Verification items for the finished model (mm, model axes). Give positions to 0.01 mm unless a question says otherwise; leave off trailing zeros. Write each loop counter-clockwise with the first axis right and the second up, starting at its lowest first coordinate (ties: lowest second). Pieces come first, ordered by that corner, then holes.
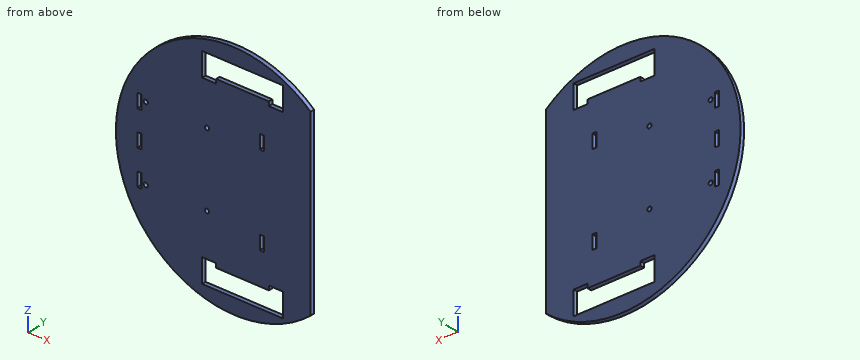
Autodesk Inventor part; units mm, degrees
ref_plane "YZ Plane" through (0, 0, 0) normal (1, 0, 0) x (0, 1, 0)
ref_plane "XZ Plane" through (0, 0, 0) normal (0, 1, 0) x (-1, 0, 0)
ref_plane "XY Plane" through (0, 0, 0) normal (0, 0, 1) x (1, 0, 0)
sketch "Sketch1" plane through (0, 0, 0) normal (0, 1, 0) x (-1, 0, 0)
  circle A0 centre (0, 0) radius 85 construction
  line L0 (-55, 64.8074) -> (-55, -64.8074) construction
  line L1 (-35, 74) -> (23, 74) construction
  line L2 (23, 74) -> (23, 60) construction
  line L3 (23, 60) -> (-35, 60) construction
  line L4 (-35, 60) -> (-35, 74) construction
  line L5 (-35, -60) -> (23, -60) construction
  line L6 (23, -60) -> (23, -74) construction
  line L7 (23, -74) -> (-35, -74) construction
  line L8 (-35, -74) -> (-35, -60) construction
  line L9 (-6, 60) -> (-6, -60)
  line L10 (6.5, 5) -> (-18.5, 5) construction
  line L11 (-18.5, 5) -> (-18.5, 57) construction
  line L12 (-18.5, 57) -> (6.5, 57) construction
  line L13 (6.5, 57) -> (6.5, 5) construction
  line L14 (6.5, 5) -> (-18.5, 57) construction
  line L15 (-18.5, 5) -> (6.5, 57) construction
  line L16 (6.5, -57) -> (-18.5, -57) construction
  line L17 (-18.5, -57) -> (-18.5, -5) construction
  line L18 (-18.5, -5) -> (6.5, -5) construction
  line L19 (6.5, -5) -> (6.5, -57) construction
  line L20 (6.5, -57) -> (-18.5, -5) construction
  line L21 (-18.5, -57) -> (6.5, -5) construction
  line L22 (66.5, -30) -> (16.5, -30) construction
  line L23 (16.5, -30) -> (16.5, 30) construction
  line L24 (16.5, 30) -> (66.5, 30) construction
  line L25 (66.5, 30) -> (66.5, -30) construction
  line L26 (66.5, -30) -> (16.5, 30) construction
  line L27 (16.5, -30) -> (66.5, 30) construction
  point P0 (-6, 31)
  point P1 (-6, -31)
  point P2 (41.5, 0)
  point P3 (-6, 0)
  point P4 (41.5, 0)
  dimension "d0" = 170
  dimension "d1" = 55
  dimension "d2" = 58
  dimension "d3" = 14
  dimension "d4" = 60
  dimension "d5" = 20
  dimension "d6" = 60
  dimension "d7" = 25
  dimension "d8" = 52
  dimension "d9" = 3
  dimension "d10" = 3
  dimension "d11" = 10
  dimension "d12" = 50
  dimension "d13" = 60
  dimension "d14" = 10
sketch "Sketch2" plane through (0, 0, 0) normal (0, 1, 0) x (-1, 0, 0)
  circle A0 centre (0, 0) radius 85 construction
  line L0 (-55, 64.8074) -> (-55, -64.8074) construction
  arc A1 (-55, -64.8074) -> (-55, 64.8074) centre (0, 0) ccw
  line L1 (-55, 64.8074) -> (-55, -64.8074)
extrude "Extrusion1" add sketch "Sketch2" along normal blind 3
sketch "Sketch3" plane through (0, 0, 0) normal (0, -1, 0) x (1, 0, 0)
  line L0 (-23, 74) -> (35, 74)
  line L1 (35, 74) -> (35, 60)
  line L2 (35, 60) -> (-23, 60)
  line L3 (-23, 60) -> (-23, 74)
  point P0 (0, 0)
extrude "Extrusion2" cut sketch "Sketch3" against normal blind 3
sketch "Sketch4" plane through (0, 0, 0) normal (0, -1, 0) x (1, 0, 0)
  line L0 (-23, 60) -> (-13, 60)
  line L1 (-13, 60) -> (-13, 57)
  line L2 (-13, 57) -> (-23, 57)
  line L3 (-23, 57) -> (-23, 60)
  line L4 (35, 60) -> (25, 60)
  line L5 (25, 60) -> (25, 57)
  line L6 (25, 57) -> (35, 57)
  line L7 (35, 57) -> (35, 60)
  point P0 (0, 0)
  dimension "d19" = 10
  dimension "d20" = 3
  dimension "d21" = 10
  dimension "d22" = 3
extrude "Extrusion3" cut sketch "Sketch4" against normal blind 3
sketch "Sketch5" plane through (0, 0, 0) normal (0, -1, 0) x (1, 0, 0)
  line L0 (18.5, 5) -> (18.5, 57) construction
  line L1 (18.5, 37) -> (21.5, 37)
  line L2 (21.5, 37) -> (21.5, 27)
  line L3 (21.5, 27) -> (18.5, 27)
  line L4 (18.5, 27) -> (18.5, 37)
  line L5 (35, 57) -> (25, 57)
  point P0 (0, 0)
  dimension "d25" = 3
  dimension "d26" = 10
  dimension "d27" = 20
extrude "Extrusion4" cut sketch "Sketch5" against normal blind 3
sketch "Sketch6" plane through (0, 0, 0) normal (0, -1, 0) x (1, 0, 0)
  line L0 (-66.5, 30) -> (-66.5, -30) construction
  line L1 (-66.5, 30) -> (-69.5, 30)
  line L2 (-69.5, 30) -> (-69.5, 20)
  line L3 (-69.5, 20) -> (-66.5, 20)
  line L4 (-66.5, 20) -> (-66.5, 30)
  line L5 (-66.5, 5) -> (-69.5, 5)
  line L6 (-69.5, 5) -> (-69.5, -5)
  line L7 (-69.5, -5) -> (-66.5, -5)
  line L8 (-66.5, -5) -> (-66.5, 5)
  line L9 (-66.5, -30) -> (-69.5, -30)
  line L10 (-69.5, -30) -> (-69.5, -20)
  line L11 (-69.5, -20) -> (-66.5, -20)
  line L12 (-66.5, -20) -> (-66.5, -30)
  point P0 (0, 0)
  point P1 (-69.5, 0)
  point P2 (-66.5, 0)
  dimension "d30" = 3
  dimension "d31" = 10
  dimension "d32" = 3
  dimension "d33" = 10
  dimension "d34" = 3
  dimension "d35" = 10
extrude "Extrusion5" cut sketch "Sketch6" against normal blind 3
sketch "Sketch7" plane through (0, 0, 0) normal (0, -1, 0) x (1, 0, 0)
  line L0 (-16.5, -30) -> (-66.5, 30) construction
  line L1 (-63.5, 26.4) -> (-19.5, 26.4)
  line L2 (-19.5, 26.4) -> (-19.5, -26.4)
  line L3 (-19.5, -26.4) -> (-63.5, -26.4)
  line L4 (-63.5, -26.4) -> (-63.5, 26.4)
  line L5 (-63.5, 26.4) -> (-19.5, -26.4) construction
  line L6 (-19.5, 26.4) -> (-63.5, -26.4) construction
  line L7 (-16.5, -30) -> (-16.5, 30) construction
  circle A0 centre (-19.5, 26.4) radius 1.5
  circle A1 centre (-19.5, -26.4) radius 1.5
  circle A2 centre (-63.5, 26.4) radius 1.5
  circle A3 centre (-63.5, -26.4) radius 1.5
  point P0 (0, 0)
  point P1 (-41.5, 0)
  dimension "d38" = 3
  dimension "d39" = 3
  dimension "d40" = 3
  dimension "d41" = 3
  dimension "d42" = 3
extrude "Extrusion6" cut sketch "Sketch7" against normal blind 3 contours L4 A2 L1 | L1 A2 L4 | A0 L2 L1 | L1 L2 A0
mirror "Mirror1" about plane through (0, 0, 0) normal (0, 0, 1) of "Extrusion2", "Extrusion3", "Extrusion4", "Extrusion6"
equation "\"d10\" = d9"
properties part number "Base Plate"
Item 1: Sectioned sample at B-B on y = 2.55. State how many separate pieces and enclosed holes the cut face has, then the cut area to 3 significant figures.
Answer key:
separate pieces: 1
enclosed holes: 11
area: 18,100 mm2
Item 2: Sectioned sample at C-C on x = 40. Record the cut outline in (y, z).
Answer key:
outline: (0, -75) - (3, -75) - (3, 75) - (0, 75) - close
Item 3: Depth check by flat-ended pin: pin 1 (1.5 mm diameter, centred on x = 32.5, y = 1, fed in from -Z); pin 2 (0.9 mm diameter, centred on x = 20.5, y = 1, fed in from +Z); pin 3 (5 mm diameter, centred on x = -8, z = 29, fed in from -Y); pin 4 (1.8 mm diameter, centred on x = -19.5, z = 26.4, fed in from -Y). Enter the tip coordinate at first touch or a pass-through.
Answer key:
pin 1: stops at z = -78.85
pin 2: stops at z = 82.6
pin 3: stops at y = 0
pin 4: passes through
Item 4: Scan lines: line 1 along Z through (x, y) = (0, 1.1); line 2 along X through (y, z) = (1.2, 26.4); line 3 along Z through (x, y) = (-19.5, 1). Record each from-to range of solid material in increasing order.
Answer key:
line 1: z = -85 to -74, -60 to 60, 74 to 85
line 2: x = -80.8 to -69.5, -66.5 to -65, -62 to -21, -18 to 55
line 3: z = -82.73 to -74, -57 to -27.9, -24.9 to 24.9, 27.9 to 57, 74 to 82.73
Item 5: Sectioned sample at A-A on x = 3.5. Record the cut outline in (y, z), then the cut area to 3 significant figures.
Answer key:
outline: (0, -84.93) - (3, -84.93) - (3, -74) - (0, -74) - close; (0, -60) - (3, -60) - (3, 60) - (0, 60) - close; (0, 74) - (3, 74) - (3, 84.93) - (0, 84.93) - close
area: 426 mm2
Item 6: Sectioned sample at D-D on z = 39.5. Record the cut outline in (x, y).
Answer key:
outline: (-75.26, 0) - (55, 0) - (55, 3) - (-75.26, 3) - close
